from build123d import *

# Parameters (mm, degrees)
SKETCH1_W           = 25
SKETCH1_H           = 3
BOSS_EXTRUDE1_DEPTH = 75
SKETCH2_R           = 1.5
BOSS_EXTRUDE2_DEPTH = 30


with BuildPart() as part:
    # Sketch1 → Boss-Extrude1 (new body)
    with BuildSketch(Plane(origin=(0, 0, 0), x_dir=(0, 0, -1), z_dir=(1, 0, 0))):
        Rectangle(SKETCH1_W, SKETCH1_H)
    extrude(amount=BOSS_EXTRUDE1_DEPTH)

    # Sketch2 → Boss-Extrude2 (add)
    with BuildSketch(Plane(origin=(75, 0, 0), x_dir=(0, 0, -1), z_dir=(1, 0, 0))):
        with Locations((-6.8, 0)):
            Circle(SKETCH2_R)
        with Locations((6.8, 0)):
            Circle(SKETCH2_R)
    extrude(amount=BOSS_EXTRUDE2_DEPTH)


solid = part.part
Could you check a few things on this model? Use its own coordinates, in mm. A direction names the side the tool comes from. Round coordinates to 2 decimals unless told otherwise and drop trailing zeros. Write each loop counter-clockwise with the first axis right and the second up, starting at its lowest first coordinate (ties: lowest second). Pieces come first, ordered by that corner, then holes. Notation, with made-up numbers: (42, 86) - (61, 86) arc R23 ccw to (61, 108) - close; hole circle Ø7 at (54, 80.25). An arc over 180 degrees is marked (long way). Use a Markdown table: item, result.
Q1. I want a section at A-A (y = 0). List the corners of the cut face in (x, z) for me.
Output values:
| item | result |
|---|---|
| outline | (0, -12.5) - (75, -12.5) - (75, -8.3) - (105, -8.3) - (105, -5.3) - (75, -5.3) - (75, 5.3) - (105, 5.3) - (105, 8.3) - (75, 8.3) - (75, 12.5) - (0, 12.5) - close |
Q2. Thinking about a two-plate mould opening in Z: for faces 3 (the flat face through (37, 0, -12.5)), 4 (the flat face through (37, 1.5, 0)), 5 (the flat face through (75, 0, 0)), which applies, released by +Z, released by -Z, zero draft, split by the parting line, or undercut?
Output values:
| item | result |
|---|---|
| face 3 | released by -Z |
| face 4 | zero draft |
| face 5 | undercut |
Q3. For faces 1 (the flat face through (37, 0, 12.5)), 2 (the cylindrical face through (89.79, 0.07, -5.3)), which set-ups out of +Z, -Z, +X, -X, +Y, -Y let a thin tool reach every point of the face, with its end or its side?
Output values:
| item | result |
|---|---|
| face 1 | +Z, +X, -X, +Y, -Y |
| face 2 | +X |
Q4. Please list where these lines run through material, in increasing order: L1, parallel to X at y = -0.4, z = -2; L2, parallel to Z at x = 78.5, y = 0.9.
Output values:
| item | result |
|---|---|
| L1 | 0 to 75 |
| L2 | -8 to -5.6, 5.6 to 8 |
Q5. I want a section at B-B (z = -10.5). List the corners of the cut face in (x, y) for me.
Output values:
| item | result |
|---|---|
| outline | (0, -1.5) - (75, -1.5) - (75, 1.5) - (0, 1.5) - close |
Q6. For pin 1 (0.9 mm diameter, centred on y = -0.5, z = -8.5, fed in from +X), with a flat end and sliding along its axis, tell me the tip position at first contact or that it passes through.
Output values:
| item | result |
|---|---|
| pin 1 | x = 105 |
